Source: CAD feature listing. Evaluate the final solid. Frame: model axes, mm. A direction names the side the tool comes from. Round coordinates to 2 decimals unless told otherwise and drop trailing zeros. Write each loop counter-clockwise with the first axis right and the second up, starting at its lowest first coordinate (ties: lowest second). Pieces come first, ordered by that corner, then holes. Notation, with made-up numbers: M 9.25,-1 L 47.25,-1 A31 cw 47.25,26 Z; hole C 13,40 d3. An arc over 180 degrees is marked long. Answer in a Markdown table with one row per item.
Autodesk Inventor part; units mm, degrees
ref_plane "Work Plane1" through (0, 4.6, -11) normal (0, 1, 0) x (-1, 0, 0)
ref_plane "YZ Plane" through (0, 0, 0) normal (1, 0, 0) x (0, 1, 0)
ref_plane "XY Plane" through (0, 0, 0) normal (0, 0, 1) x (1, 0, 0)
sketch "Sketch1" plane through (0, 0, 0) normal (0, 0, 1) x (1, 0, 0)
  circle A0 centre (0, 0) radius 5.1
  line L0 (-8.25, 8.25) -> (8.25, 8.25)
  line L1 (8.25, 8.25) -> (8.25, -8.25)
  line L2 (8.25, -8.25) -> (-8.25, -8.25)
  line L3 (-8.25, -8.25) -> (-8.25, 8.25)
  line L4 (-8.25, 8.25) -> (8.25, -8.25) construction
  line L5 (8.25, 8.25) -> (-8.25, -8.25) construction
  line L6 (0.75, -8.25) -> (-0.75, -8.25)
  line L7 (-0.75, -8.25) -> (-0.75, 8.25)
  line L8 (-0.75, 8.25) -> (0.75, 8.25)
  line L9 (0.75, 8.25) -> (0.75, -8.25)
  line L10 (0.75, -8.25) -> (-0.75, 8.25) construction
  line L11 (-0.75, -8.25) -> (0.75, 8.25) construction
  line L12 (8.25, 0.75) -> (-8.25, 0.75)
  line L13 (-8.25, 0.75) -> (-8.25, -0.75)
  line L14 (-8.25, -0.75) -> (8.25, -0.75)
  line L15 (8.25, -0.75) -> (8.25, 0.75)
  line L16 (8.25, 0.75) -> (-8.25, -0.75) construction
  line L17 (-8.25, 0.75) -> (8.25, -0.75) construction
  point P0 (0.75, -5.0446)
  point P1 (5.0446, -0.75)
  point P2 (5.0446, 0.75)
  point P3 (0.75, 5.0446)
  point P4 (-0.75, 5.0446)
  point P5 (-5.0446, 0.75)
  point P6 (-5.0446, -0.75)
  point P7 (-0.75, -5.0446)
  dimension "d0" = 10.2
  dimension "d1" = 16.5
  dimension "d2" = 1.5
  dimension "d3" = 1.5
  dimension "d38" = 16.5
extrude "Extrusion1" add sketch "Sketch1" against normal blind 11
extrude "Extrusion2" cut sketch "Sketch1" against normal blind 7 contours A0 L14 L9 L12 | A0 L12 L1 L14 | L12 L9 A0 | A0 L9 L14 | L9 L12 L7 A0 | A0 L7 L0 L9 | L9 L14 L7 L12 | L9 L2 L7 A0 | A0 L7 L14 L9 | L7 L12 A0 | L7 L14 A0 L12 | A0 L14 L7 | A0 L14 L3 L12
sketch "Sketch2" plane through (0, 0, -11) normal (0, 0, -1) x (-1, 0, 0)
  circle A0 centre (0, 0) radius 5
  dimension "d8" = 10
extrude "Extrusion3" [suppressed]
fillet "Fillet1" radius 6 4 edges at (8.25, 8.25, -5.5) (8.25, -8.25, -5.5) (-8.25, -8.25, -5.5) (-8.25, 8.25, -5.5)
sketch "Sketch3" plane through (0, 0, -26) normal (0, 0, -1) x (-1, 0, 0)
  line L0 (4, 2.7238) -> (10.2, 2.7238)
  line L1 (10.2, 2.7238) -> (10.2, -2.0551)
  line L2 (10.2, -2.0551) -> (4, -2.0551)
  line L3 (4, -2.0551) -> (4, 2.7238)
  arc A0 (2.5948, 0.1645) -> (2.1, -1.533) centre (0, 0) ccw
  circle A1 centre (0, 0) radius 5
  line L4 (0, 5) -> (10.2, 5)
  line L5 (10.2, 5) -> (10.2, -5)
  line L6 (10.2, -5) -> (0, -5)
  arc A2 (8.25, 2.25) -> (2.25, 8.25) centre (2.25, 2.25) ccw
  line L7 (2.25, 8.25) -> (-2.25, 8.25)
  arc A3 (-2.25, 8.25) -> (-8.25, 2.25) centre (-2.25, 2.25) ccw
  line L8 (-8.25, 2.25) -> (-8.25, -2.25)
  arc A4 (-8.25, -2.25) -> (-2.25, -8.25) centre (-2.25, -2.25) ccw
  line L9 (-2.25, -8.25) -> (2.25, -8.25)
  arc A5 (2.25, -8.25) -> (8.25, -2.25) centre (2.25, -2.25) ccw
  line L10 (8.25, -2.25) -> (8.25, 2.25)
  line L11 (-2.6, -2.9034) -> (-2.6, 2.8378)
  circle A6 centre (0, 0) radius 2.6
  point P0 (0.75, 5.0446)
  point P1 (2.1, -1.533)
  point P2 (2.5948, 0.1645)
  dimension "d12" = 6.2
  dimension "d13" = 4
  dimension "d14" = 5.2
extrude "Extrusion4" [suppressed]
sketch "Sketch4" plane through (-10.2, -5, -26) normal (-1, 0, 0) x (0, 0, 1)
  circle A0 centre (4, 5) radius 1.7
  line L0 (0, 0) -> (0, 10)
  point P0 (26, 5)
  point P1 (0, 5)
  point P2 (0, 5)
  dimension "d17" = 3.4
  dimension "d18" = 4
extrude "Extrusion5" [suppressed]
extrude "Extrusion6" [suppressed]
fillet "Fillet2" [suppressed]
fillet "Fillet3" [suppressed]
sketch "Sketch5" plane through (0, 0, -11) normal (0, 0, -1) x (-1, 0, 0)
  arc A0 (8.25, 2.25) -> (2.25, 8.25) centre (2.25, 2.25) ccw
  line L0 (2.25, 8.25) -> (-2.25, 8.25)
  arc A1 (-2.25, 8.25) -> (-8.25, 2.25) centre (-2.25, 2.25) ccw
  line L1 (-8.25, 2.25) -> (-8.25, -2.25)
  arc A2 (-8.25, -2.25) -> (-2.25, -8.25) centre (-2.25, -2.25) ccw
  line L2 (-2.25, -8.25) -> (2.25, -8.25)
  arc A3 (2.25, -8.25) -> (8.25, -2.25) centre (2.25, -2.25) ccw
  line L3 (8.25, -2.25) -> (8.25, 2.25)
  line L4 (-5.5, 5.5) -> (5.5, 5.5)
  line L5 (5.5, 5.5) -> (5.5, -5.5)
  line L6 (5.5, -5.5) -> (-5.5, -5.5)
  line L7 (-5.5, -5.5) -> (-5.5, 5.5)
  line L8 (-5.5, 5.5) -> (5.5, -5.5) construction
  line L9 (5.5, 5.5) -> (-5.5, -5.5) construction
  point P0 (0, 0)
  dimension "d31" = 11
  dimension "d32" = 11
extrude "Extrusion7" [suppressed]
sketch "Sketch6" plane through (0, 0, -7) normal (0, 0, 1) x (1, 0, 0)
  circle A0 centre (0, 0) radius 5.1
extrude "Extrusion8" cut sketch "Sketch6" against normal blind 2
sketch "Sketch7" plane through (0, 0, -11) normal (0, 0, -1) x (-1, 0, 0)
  circle A0 centre (0, 0) radius 4.6
  circle A1 centre (0, 0) radius 2.7
  dimension "d35" = 9.2
  dimension "d39" = 5.4
extrude "Extrusion9" add sketch "Sketch7" along normal blind 17.94
ref_plane "Work Plane1" through (0, 4.6, -11) normal (0, 1, 0) x (-1, 0, 0)
sketch "Sketch8" plane through (0, 4.6, -11) normal (0, 1, 0) x (-1, 0, 0)
  line L0 (2.7, -17.94) -> (-2.7, -17.94)
  line L1 (-2.7, -17.94) -> (-2.7, -14.94)
  line L2 (-2.7, -14.94) -> (2.7, -14.94)
  line L3 (2.7, -14.94) -> (2.7, -17.94)
  line L4 (-4.6, -17.94) -> (4.6, -17.94)
  point P0 (0, 11)
  point P1 (0, -17.94)
  dimension "d40" = 5.4
  dimension "d41" = 3
sketch "Sketch9" plane through (0, 0, -28.94) normal (0, 0, -1) x (-1, 0, 0)
  line L0 (2.7, 4.6) -> (-2.7, 4.6)
  line L1 (-2.7, 4.6) -> (2.7, 4.6)
  line L2 (2.7, 4.6) -> (2.7, 7.1)
  line L3 (2.7, 7.1) -> (-2.7, 7.1)
  line L4 (-2.7, 7.1) -> (-2.7, 4.6)
  line L5 (-4.2, 4.6) -> (4.2, 4.6)
  line L6 (4.2, 4.6) -> (4.2, 8.6)
  line L7 (4.2, 8.6) -> (-4.2, 8.6)
  line L8 (-4.2, 8.6) -> (-4.2, 4.6)
  line L9 (-4.2, 4.6) -> (-4.2, 1.8762)
  circle A0 centre (0, 0) radius 4.6
  line L10 (4.2, 4.6) -> (4.2, 1.8762)
  point P0 (0, 4.6)
  dimension "d42" = 5.4
  dimension "d43" = 2.5
  dimension "d44" = 1.5
  dimension "d45" = 1.5
  dimension "d46" = 1.5
extrude "Extrusion10" add sketch "Sketch9" against normal blind 4 contours L5 L10 A0 L0 | L2 L3 L4 L5 L8 L7 L6 | A0 L9 L5 L0
sketch "Sketch10" plane through (-4.2, 8.6, -28.94) normal (0, 1, 0) x (1, 0, 0)
  line L0 (4.2, -4) -> (4.2, 0)
  circle A0 centre (4.2, -2) radius 1.6
  point P0 (4.2, -28.94)
  dimension "d49" = 3.2
extrude "Extrusion11" cut sketch "Sketch10" against normal blind 9.25
sketch "Sketch11" plane through (0, 0, -11) normal (0, 0, -1) x (-1, 0, 0)
  circle A0 centre (0, 0) radius 2.7
extrude "Extrusion12" add sketch "Sketch11" along normal blind 1
properties part number "rubik_adapter"
Q1. Section B-B (y = 0). Return loops of the section in (x, z), and give its area (3 significant figures).
Solutions:
| item | result |
|---|---|
| outline | M -8.25,-11 L -4.6,-11 L -4.6,-28.94 L -2.7,-28.94 L -2.7,-12 L 2.7,-12 L 2.7,-28.94 L 4.6,-28.94 L 4.6,-11 L 8.25,-11 L 8.25,-7 L 5.1,-7 L 5.1,-9 L -5.1,-9 L -5.1,-7 L -8.25,-7 Z |
| area | 119 mm2 |
Q2. Section C-C (y = 3). Return loops of the section in (x, z), and give its area (3 significant figures).
Solutions:
| item | result |
|---|---|
| outline | M -8.2,-11 L -3.49,-11 L -3.49,-24.94 L -4.2,-24.94 L -4.2,-28.94 L 4.2,-28.94 L 4.2,-24.94 L 3.49,-24.94 L 3.49,-11 L 8.2,-11 L 8.2,0 L 4.12,0 L 4.12,-9 L -4.12,-9 L -4.12,0 L -8.2,0 Z; hole C 0,-26.94 d3.2 |
| area | 229 mm2 |
Q3. Pull-direction query (Y, two-part tool) for faces 1 (the flat face through (-1, 8.25, -5)), 2 (the flat face through (7, 0.75, -3)), 3 (the flat face through (0, 7, -7)); classes: pulls with the +Y half, pulls with the -Y half, needs draft (parallel to the pull), parting line crosses it, or undercut.
Solutions:
| item | result |
|---|---|
| face 1 | pulls with the +Y half |
| face 2 | undercut |
| face 3 | needs draft |
Q4. Contact query for flat-ended pins moving along their axis: pin 1 Ø3 at (x, y) = (-2, -0.5) entering from +Z; pin 2 Ø6 at (y, z) = (-6.5, -8) entering from -X; pin 3 Ø2.5 at (y, z) = (-6.5, -2.5) entering from -X. Output: stop coordinate, or through.
Solutions:
| item | result |
|---|---|
| pin 1 | stops at z = -9 |
| pin 2 | stops at x = -8.12 |
| pin 3 | stops at x = -7.45 |
Q5. Section A-A (z = -6). Return loops of the section in (x, y), and give its area (3 significant figures).
Solutions:
| item | result |
|---|---|
| outline | M -8.25,-2.25 A6 ccw -2.25,-8.25 L -0.75,-8.25 L -0.75,-5.04 A5.1 cw -5.04,-0.75 L -8.25,-0.75 Z; M -8.25,0.75 L -5.04,0.75 A5.1 cw -0.75,5.04 L -0.75,8.25 L -2.25,8.25 A6 ccw -8.25,2.25 Z; M 0.75,-8.25 L 2.25,-8.25 A6 ccw 8.25,-2.25 L 8.25,-0.75 L 5.04,-0.75 A5.1 cw 0.75,-5.04 Z; M 0.75,5.04 A5.1 cw 5.04,0.75 L 8.25,0.75 L 8.25,2.25 A6 ccw 2.25,8.25 L 0.75,8.25 Z |
| area | 141 mm2 |
Q6. Material intervals for probe 1 along X at (y, z) = (3.3, -26.94); probe 2 along Y at (x, z) = (0.25, -8); probe 3 along Z at (x, y) = (6, 6.75), sorted ascending.
Solutions:
| item | result |
|---|---|
| probe 1 | x = -4.2 to -1.6, 1.6 to 4.2 |
| probe 2 | y = -8.25 to -5.09, 5.09 to 8.25 |
| probe 3 | z = -11 to 0 |
Q7. Access query for faces 4 (the flat face through (4.2, 5, -27)), 5 (the flat face through (7, 0, -7)), 6 (the flat face through (0.75, -7, -3)), 7 (the cylindrical face through (0.351, -2.677, -20.351)). Directions: +Z, -Z, +X, -X, +Y, -Y. A direction counts if a zero-diameter tool reaches every point of the face in a straight line with its end or side. Return the directions, or none.
Solutions:
| item | result |
|---|---|
| face 4 | -Z, +X, +Y |
| face 5 | +Z, +X, -X |
| face 6 | +Z, +Y, -Y |
| face 7 | -Z |
Q8. Section D-D (x = -5.5). Return loops of the section in (y, z).
Solutions:
| item | result |
|---|---|
| outline | M -7.29,-11 L 7.29,-11 L 7.29,0 L 0.75,0 L 0.75,-7 L -0.75,-7 L -0.75,0 L -7.29,0 Z |
